Source: three-view drawing plus pictorial views. Frame: mm from the lowest corner of the part. Give positions to 0.01 mm unless a question says otherwise; leave off trailing zeros. Order: outer loops, then holes, each group sorted by start corner. A loop starts at its lowest first (then second) coordinate and runs counter-clockwise, first axis right, second up. Notation, with made-up numbers: M 34,15.25 L 39,15.25 A27 ccw 39,40.25 Z; hole C -23,81.5 d4. An arc over 180 degrees is marked long. Use CSV: the item, a comma, the result in double quotes. Start each with the question number.
Item 1: Section query C-C on x = 111. Return loops of the section in (y, z).
Item 2: First-contact query: pin 1 (9 mm diameter, centred on x = 69.5, y = 9.5, fed in from +Z); pin 2 (1.5 mm diameter, centred on y = 13, z = 2, fed in from -X). Flat tips, straight axial feed; report the tip coordinate or a pass-through.
Item 3: Section query B-B on z = 1.1. Count the separate pieces of the cut face and the enclosed holes in it, and give its area (3 significant figures).
Item 4: Section query A-A on x = 89.5. Return loops of the section in (y, z).
Item 5: Ray query, probe 1 along Z at (x, y) = (141, 15); probe 2 along Y at (x, z) = (131, 3.45); probe 3 along Y at (x, z) = (109.5, 3.15). Return the intervals inside material, ascending. Write a range as from..to.
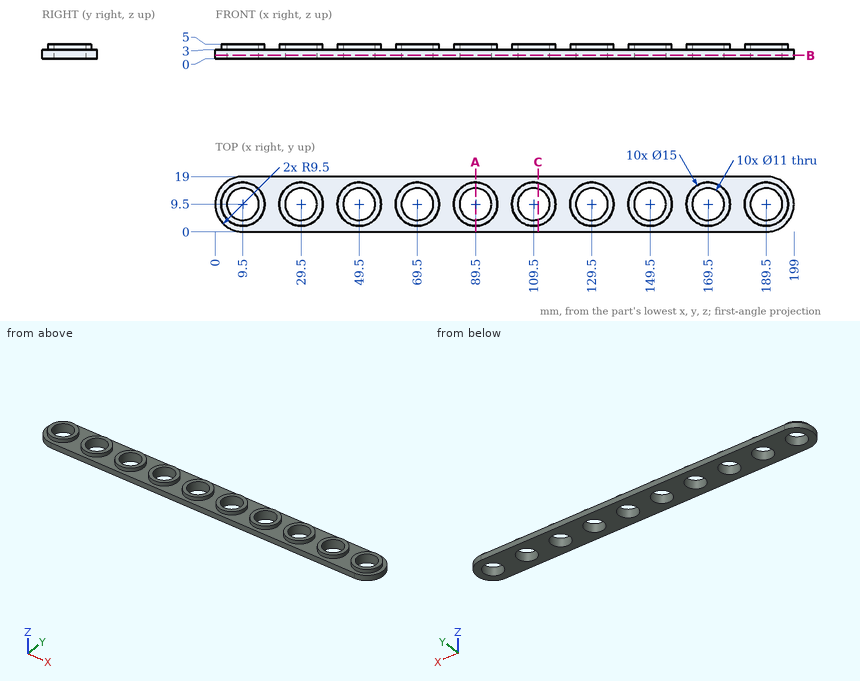
Verdict:
1,outline,"M 0,0 L 4.21,0 L 4.21,5 L 2.15,5 L 2.15,3 L 0,3 Z; M 14.79,0 L 19,0 L 19,3 L 16.85,3 L 16.85,5 L 14.79,5 Z"
2,pin 1,"through"
2,pin 2,"x = 0.41"
3,separate pieces,"1"
3,enclosed holes,"10"
3,area,"2,750 mm2"
4,outline,"M 0,0 L 4,0 L 4,5 L 2,5 L 2,3 L 0,3 Z; M 15,0 L 19,0 L 19,3 L 17,3 L 17,5 L 15,5 Z"
5,probe 1,"0..3"
5,probe 2,"2.15..4.21, 14.79..16.85"
5,probe 3,"2..4, 15..17"
